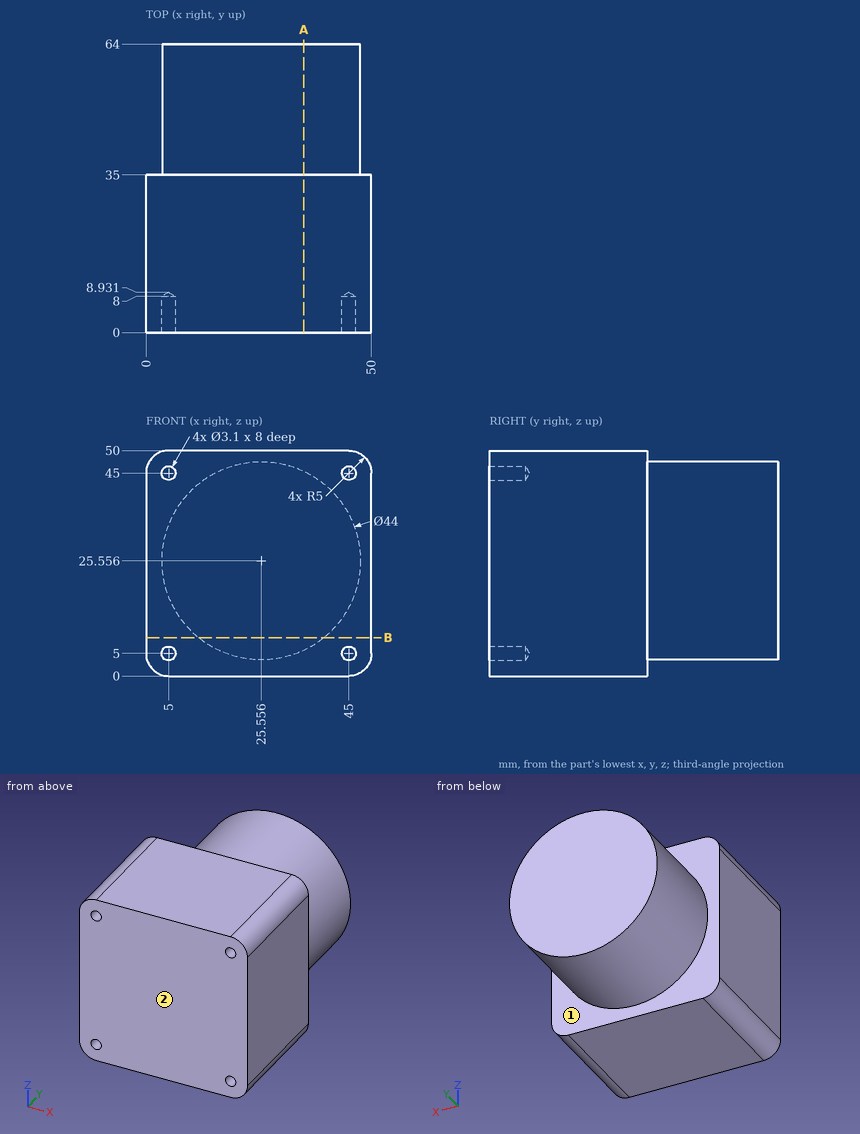
Design review of the part shown in the three views and the two pictorial views. Dimensions are in mm from the part's minimum x, y and z. A direction names the side the tool comes from. Round coordinates to 2 decimals unless told otherwise and drop trailing zeros. Order: outer loops, then holes, each group sorted by start corner. A loop starts at its lowest first (then second) coordinate and runs counter-clockwise, first axis right, second up.
Item 1: Add section A-A, the plane x = 35. State the section outline as (y, z) points (1 decimal).
Working result:
outline: (0, 0) - (35, 0) - (35, 5.7) - (64, 5.7) - (64, 45.4) - (35, 45.4) - (35, 50) - (0, 50) - close
Item 2: Add section B-B, the plane z = 8.5. State the section outline as (x, y) points.
Working result:
outline: (0, 0) - (50, 0) - (50, 35) - (39.45, 35) - (39.45, 64) - (11.66, 64) - (11.66, 35) - (0, 35) - close
Item 3: Machinability: for the marked faces 1 and 2, which of the approach directions +Z, -Z, +X, -X, +Y, -Y give a long, thin tool a straight path to every point of the face, cutting with its end or side? Answer none if there is none.
Working result:
face 1: +Y
face 2: +Z, -Z, +X, -X, -Y
Item 4: For pin 1 (2.5 mm diameter, centred on x = 5, z = 45, fed in from +Y), flat-tipped, find the tip position at first contact; note if it passes through.
Working result:
pin 1: stops at y = 35
Item 5: To check wall thickness, follow probe 1 along Z at (x, y) = (45, 2); probe 2 along Y at (x, z) = (7, 37.5). State the ranges of each line that lie inside material, in increasing order.
Working result:
probe 1: z = 0 to 3.45, 6.55 to 43.45, 46.55 to 50
probe 2: y = 0 to 35
